Source: CAD feature listing. Evaluate the final solid. Frame: model axes, mm. A direction names the side the tool comes from. Coordinates: 2 decimals unless noted, no trailing zeros. Order: outer loops, then holes, each group sorted by start corner. A loop starts at its lowest first (then second) coordinate and runs counter-clockwise, first axis right, second up.
Item 1: Reachability of faces 1 (the flat face through (0, 1, 1)), 2 (the flat face through (0, 2, 0)) from +Z, -Z, +X, -X, +Y, -Y: full face, straight path, thin tool, end or side. Return the list, or none.
Item 2: Mould query, pull axis X, two halves, no side actions, for faces 3 (the conical face through (0.1, 0, 0)), 4 (the flat face through (-0.87, 0.49, 1.06)), 5 (the flat face through (0, 0, -16)), 6 (the cylindrical face through (-1.5, 0.07, -7.8)). Classes: released by +X, released by -X, zero draft, split by the parting line, or undercut.
Item 3: Ray query, line 1 (Z direction, x = 2.5, y = -0.5); line 2 (Z direction, x = 1.5, y = 1.6); line 3 (Y direction, x = -0.1, z = -3). Return the intervals inside material, ascending.
Item 4: Section A-A on z = -9.5. Return the cut outline in (x, y), then the cut area to 3 significant figures.
Item 5: Contact query for flat-ended pins moving along their axis: P1, Ø1, axis at y = -1.5, z = -5.5, coming from the +X side; P2, Ø0.9, axis at x = 0, z = 1, coming from the -Y side. Output: stop coordinate, or through.
Solid Edge part; units mm, degrees
sketch "Sketch1" plane through (0, 0, 0) normal (0, -1, 0) x (1, 0, 0)
  line L0 (0, -16) -> (1.5, -16)
  line L1 (1.5, -16) -> (1.5, -0.115)
  arc A0 (1.5, -0.105) -> (1.5, -0.115) centre (1.5038, -0.11) ccw
  line L2 (1.5, -0.105) -> (1.5, 0)
  line L3 (1.5, 0) -> (2.85, 0)
  line L4 (2.85, 0) -> (2.85, 0.165)
  arc A1 (1.27, 1.65) -> (2.85, 0.165) centre (-0.3628, -1.6703) cw
  line L5 (0, 1.65) -> (1.27, 1.65)
  dimension "D1" = 1.5
revolve "RevolvedProtrusion1" add sketch "Sketch1" angle 360 about axis through (0, 0, 5) along (0, 0, -1)
sketch "Sketch2" plane through (0, 0, 0) normal (0, -1, 0) x (1, 0, 0)
  line L0 (0, -0.0566) -> (1.1545, 0.61)
  line L1 (1.1545, 0.61) -> (1.1545, 1.65)
  line L2 (1.1545, 1.65) -> (0, 1.65)
revolve "RevolvedCutout1" cut sketch "Sketch2" angle 360 about axis through (0, 0, 5.3) along (0, 0, -1)
sketch "Sketch3" plane through (0, 0, 0) normal (0, 0, -1) x (0, 1, 0)
  arc A0 (-1, 0.577) -> (-1, -0.577) centre (0, 0) ccw
  line L0 (-1, 0.577) -> (-1, -0.577)
extrude "Protrusion1" add sketch "Sketch3" against normal blind 1.65
pattern_circular "Pattern1" count 6 over 360 about axis through (0, 0, 0) along (0, 0, -1) of "Protrusion1"
fillet "Round_1" radius 0.185 1 edges at (-1.27, 0, 1.65)
sketch "Sketch4" plane through (0, 0, 0) normal (0, -1, 0) x (1, 0, 0)
  line L0 (0, 0.9501) -> (1.2122, 1.65)
  line L1 (1.2122, 1.65) -> (0, 1.65)
revolve "RevolvedCutout2" cut sketch "Sketch4" angle 360 about axis through (0, 0, 5.3) along (0, 0, -1)
sketch "Sketch5" plane through (0, 0, 0) normal (0, -1, 0) x (1, 0, 0)
  line L0 (-1.5, 0) -> (-1.5, -0.1)
  line L1 (-1.6, 0) -> (-1.5, 0)
  arc A0 (-1.6, 0) -> (-1.5, -0.1) centre (-1.6, -0.1) cw
revolve "RevolvedProtrusion2" add sketch "Sketch5" angle 360 about axis through (0, 0, -0.5) along (0, 0, 1)
cosmetic_thread "Thread1"
chamfer "Chamfer1" distance 0.3065 angle 45 1 edges at (-1.5, 0, -16)
properties material "Stahl"
Answer list:
1. face 1: +Z
1. face 2: -Z
2. face 3: undercut
2. face 4: undercut
2. face 5: zero draft
2. face 6: split by the parting line
3. line 1: z = 0 to 0.61
3. line 2: z = 0 to 1
3. line 3: y = -1.5 to 1.5
4. outline: circle Ø3 at (0, 0)
4. area: 7.07 mm2
5. P1: stops at x = 1.12
5. P2: stops at y = -2.6
